The model under review builds one solid part; all positions refer to its coordinate system, in mm. Give positions to 0.01 mm unless a question says otherwise; leave off trailing zeros. Order: outer loops, then holes, each group sorted by start corner. A loop starts at its lowest first (then second) coordinate and runs counter-clockwise, first axis right, second up. Notation, with made-up numbers: (-14, 26.5) - (36, 26.5) arc R20 cw to (36, 39.5) - close; hole circle Ø6 at (-31, -38.75). An arc over 180 degrees is marked (long way). Use CSV: the item, a comma, the result in double quotes.
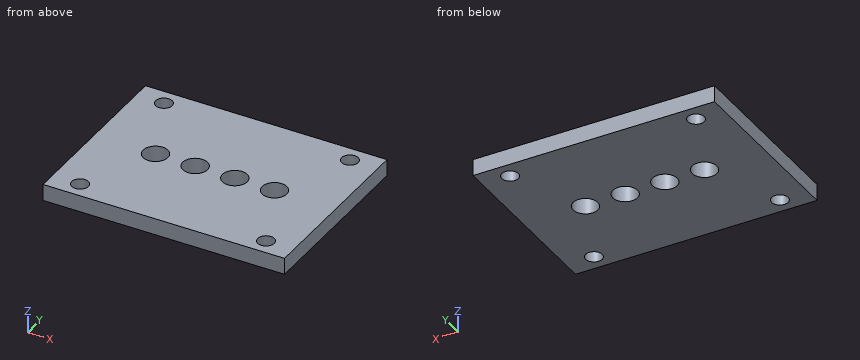
```python
from build123d import *

# Parameters (mm, degrees)
SKETCH1_W           = 185.547
SKETCH1_H           = 139.7
BOSS_EXTRUDE1_DEPTH = 12.7
SKETCH2_R           = 9.525
CUT_EXTRUDE1_DEPTH  = 117.821379902
SKETCH3_R           = 6.35
CUT_EXTRUDE2_DEPTH  = 12.7


with BuildPart() as part:
    # Sketch1 → Boss-Extrude1 (new body)
    with BuildSketch(Plane.XY):
        Rectangle(SKETCH1_W, SKETCH1_H)
    extrude(amount=BOSS_EXTRUDE1_DEPTH)

    # Sketch2 → Cut-Extrude1 (cut, through all)
    with BuildSketch(Plane.XY.offset(12.7)):
        with Locations((-45.72, 0)):
            Circle(SKETCH2_R)
        with Locations((-15.24, 0)):
            Circle(SKETCH2_R)
        with Locations((15.24, 0)):
            Circle(SKETCH2_R)
        with Locations((45.72, 0)):
            Circle(SKETCH2_R)
    extrude(amount=-CUT_EXTRUDE1_DEPTH, mode=Mode.SUBTRACT)

    # Sketch3 → Cut-Extrude2 (cut)
    with BuildSketch(Plane.XY.offset(12.7)):
        with Locations((-71.4375, 57.15)):
            Circle(SKETCH3_R)
        with Locations((-71.4375, -57.15)):
            Circle(SKETCH3_R)
        with Locations((71.4375, 57.15)):
            Circle(SKETCH3_R)
        with Locations((71.4375, -57.15)):
            Circle(SKETCH3_R)
    extrude(amount=-CUT_EXTRUDE2_DEPTH, mode=Mode.SUBTRACT)


solid = part.part
```
Item 1: Take a section at B-B, the plane x = 45.72. Give the boundary of the cut face in (y, z) (3 decimals), and give its area (3 significant figures).
Results list:
outline,"(-69.85, 0) - (-9.525, 0) - (-9.525, 12.7) - (-69.85, 12.7) - close; (9.525, 0) - (69.85, 0) - (69.85, 12.7) - (9.525, 12.7) - close"
area,"1,530 mm2"
Item 2: Take a section at D-D, the plane x = -68. Give the boundary of the cut face in (y, z).
Results list:
outline,"(-69.85, 0) - (-62.49, 0) - (-62.49, 12.7) - (-69.85, 12.7) - close; (-51.81, 0) - (51.81, 0) - (51.81, 12.7) - (-51.81, 12.7) - close; (62.49, 0) - (69.85, 0) - (69.85, 12.7) - (62.49, 12.7) - close"
Item 3: Wall thickness on L1, parallel to Y at x = -75.5, z = 11.25; L2, parallel to X at y = -61, z = 3.75; L3, parallel to Y at x = 45.5, z = 5: over which ranges is each line inside the solid? List them lowest first.
Results list:
L1,"y = -69.85 to -62.03, -52.27 to 52.27, 62.03 to 69.85"
L2,"x = -92.77 to -76.49, -66.39 to 66.39, 76.49 to 92.77"
L3,"y = -69.85 to -9.52, 9.52 to 69.85"
Item 4: Take a section at A-A, the plane y = -57.15. Give the boundary of the cut face in (x, z), and give its area (3 significant figures).
Results list:
outline,"(-92.77, 0) - (-77.79, 0) - (-77.79, 12.7) - (-92.77, 12.7) - close; (-65.09, 0) - (65.09, 0) - (65.09, 12.7) - (-65.09, 12.7) - close; (77.79, 0) - (92.77, 0) - (92.77, 12.7) - (77.79, 12.7) - close"
area,"2,030 mm2"
Item 5: Take a section at C-C, the plane z = 3. State how many separate pieces and enclosed holes the cut face has, and give its area (3 significant figures).
Results list:
separate pieces,"1"
enclosed holes,"8"
area,"24,300 mm2"
Item 6: Clearance check with a flat-ended pin moving along its axis: pin 1 (7.5 mm diameter, centred on x = -71.44, y = -57.15, fed in from +Z). State where the tip first meets the part, or that it passes through.
Results list:
pin 1,"passes through"
